Work out the finished part from the listing and answer in its coordinate system (mm). A direction names the side the tool comes from. Give positions to 0.01 mm unless a question says otherwise; leave off trailing zeros. Loops run counter-clockwise (first coordinate to the right, second up) from the corner with the lowest first, then second, coordinate; pieces in that order, holes last. Notation, with made-up numbers: (-31.75, 0.5) - (2.25, 0.5) arc R21 ccw to (2.25, 36.5) - close; hole circle Ø8 at (56, -16.75). An arc over 180 degrees is marked (long way). One line per item, written item: value.
from build123d import *

# Parameters (mm, degrees)
SKETCH1_R           = 12.5
BOSS_EXTRUDE1_DEPTH = 3
SKETCH2_R           = 12.5
SKETCH2_R_2         = 3.05
BOSS_EXTRUDE2_DEPTH = 2


with BuildPart() as part:
    # Sketch1 → Boss-Extrude1 (new body)
    with BuildSketch(Plane(origin=(0, 0, 0), x_dir=(1, 0, 0), z_dir=(0, 1, 0))):
        with Locations(Location((0, 0, 0), (0, 0, 270))):
            Circle(SKETCH1_R)
        Polygon((9.93042463, 0), (4.965212315, 8.6), (-4.965212315, 8.6), (-9.93042463, 0), (-4.965212315, -8.6), (4.965212315, -8.6), align=None, mode=Mode.SUBTRACT)
    extrude(amount=BOSS_EXTRUDE1_DEPTH)

    # Sketch2 → Boss-Extrude2 (add)
    with BuildSketch(Plane(origin=(0, 3, 0), x_dir=(1, 0, 0), z_dir=(0, 1, 0))):
        with Locations(Location((0, 0, 0), (0, 0, 270))):
            Circle(SKETCH2_R)
        with Locations(Location((0, 0, 0), (0, 0, 270))):
            Circle(SKETCH2_R_2, mode=Mode.SUBTRACT)
    extrude(amount=BOSS_EXTRUDE2_DEPTH)


solid = part.part
1. For faces 4 (the flat face through (0, 3, -4)), 5 (the flat face through (-3, 5, 3)), determine the directions among +Z, -Z, +X, -X, +Y, -Y from which every point of the face is accessible in a straight line to the end or side of a thin tool.
Output:
face 4: -Y
face 5: +Z, -Z, +X, -X, +Y
2. Section C-C (z = 2.5) is taken. Write down the section's boundary in (x, y).
Output:
outline: (-12.25, 0) - (-8.49, 0) - (-8.49, 3) - (-1.75, 3) - (-1.75, 5) - (-12.25, 5) - close; (1.75, 3) - (8.49, 3) - (8.49, 0) - (12.25, 0) - (12.25, 5) - (1.75, 5) - close
3. Section A-A (y = 1.3) is taken. Write down the section's boundary in (x, z), and give its area (3 significant figures).
Output:
outline: circle Ø25 at (0, 0); hole (-9.93, 0) - (-4.97, -8.6) - (4.97, -8.6) - (9.93, 0) - (4.97, 8.6) - (-4.97, 8.6) - close
area: 235 mm²
4. Find the intervals of material crossed by line 1 along X through (y, z) = (4.35, 0); line 2 along Y through (x, z) = (6.25, -3.5); line 3 along X through (y, z) = (0.55, -3.25), in increasing order.
Output:
line 1: x = -12.5 to -3.05, 3.05 to 12.5
line 2: y = 3 to 5
line 3: x = -12.07 to -8.05, 8.05 to 12.07
5. The mould has two halves that part along Z. Classify faces 1 (the flat face through (-7.483, 1.479, 4.24)), 2 (the flat face through (9, 0, 3)), 3 (the cylindrical face through (3.755, 2.465, 11.923)): released by +Z, released by -Z, zero draft, split by the parting line, or undercut.
Output:
face 1: undercut
face 2: zero draft
face 3: split by the parting line
6. Flat-ended cylindrical pins translate along their axes: pin 1 Ø1 at (y, z) = (1, -2) entering from -X; pin 2 Ø6 at (x, z) = (-6.5, 9.5) entering from -Y; pin 3 Ø1.5 at (x, y) = (-1, 1.5) entering from -Z; pin 4 Ø1.5 at (x, y) = (-9.5, 1) entering from +Z. Find the tip coordinate at first contact, or state that the pin passes through.
Output:
pin 1: stops at x = -12.41
pin 2: stops at y = 0
pin 3: stops at z = -12.5
pin 4: stops at z = 8.93
7. Section D-D (z = -7.25) is taken. Write down the section's boundary in (x, y), and give its area (3 significant figures).
Output:
outline: (-10.18, 0) - (-5.74, 0) - (-5.74, 3) - (5.74, 3) - (5.74, 0) - (10.18, 0) - (10.18, 5) - (-10.18, 5) - close
area: 67.4 mm²
8. Section B-B (x = 0) is taken. Write down the section's boundary in (y, z), and give its area (3 significant figures).
Output:
outline: (0, -12.5) - (5, -12.5) - (5, -3.05) - (3, -3.05) - (3, -8.6) - (0, -8.6) - close; (0, 8.6) - (3, 8.6) - (3, 3.05) - (5, 3.05) - (5, 12.5) - (0, 12.5) - close
area: 61.2 mm²
